Here's how the part is built. I have some questions about the finished solid (model axes, mm). Coordinates: 2 decimals unless noted, no trailing zeros. Loops run counter-clockwise (first coordinate to the right, second up) from the corner with the lowest first, then second, coordinate; pieces in that order, holes last. Notation, with made-up numbers: (44.5, 71.5) -> (90.5, 71.5) arc R18 cw to (90.5, 84.5) -> close; hole circle Ø9 at (-9, 27). An arc over 180 degrees is marked (long way). Use CSV: the item, a comma, the result in double quotes. Start each with the question number.
from build123d import *

# Parameters (mm, degrees)
SKETCH1_R           = 6.5
BOSS_EXTRUDE1_DEPTH = 4
SKETCH5_R           = 1.5
CUT_EXTRUDE1_DEPTH  = 4


with BuildPart() as part:
    # Sketch1 → Boss-Extrude1 (new body)
    with BuildSketch(Plane.XY):
        Circle(SKETCH1_R)
    extrude(amount=BOSS_EXTRUDE1_DEPTH)

    # Sketch4 → Cut-Revolve1 (revolve, cut)
    with BuildSketch(Plane(origin=(0, 0, 0), x_dir=(0, -1, 0), z_dir=(1, 0, 0)), mode=Mode.PRIVATE) as cut_revolve1_sk:
        with BuildLine():
            Line((6.5, -1), (6.5, -3))
            ThreePointArc((6.5, -3), (5.5, -2), (6.5, -1))
        make_face()
    revolve(cut_revolve1_sk.sketch.rotate(Axis((0, 0, 0), (0, 0, 1)), 270), axis=Axis((0, 0, 0), (0, 0, 1)), mode=Mode.SUBTRACT)

    # Sketch5 → Cut-Extrude1 (cut)
    with BuildSketch(Plane(origin=(0, 0, 0), x_dir=(-1, 0, 0), z_dir=(0, 0, -1))):
        Circle(SKETCH5_R)
    extrude(amount=-CUT_EXTRUDE1_DEPTH, mode=Mode.SUBTRACT)


solid = part.part
1) Thinking about a two-plate mould opening in Y: for faces 1 (the face through (0, 2, 4)), 2 (the face through (1.5, 0.07, 1.97)), 3 (the face through (-5.158, -3.955, 3.493)), which applies, pulls with the +Y half, pulls with the -Y half, needs draft (parallel to the pull), parting line crosses it, or undercut?
2) Please list where these lines run through material, in increasing order: L1, parallel to Z at x = 5, y = -3.25; L2, parallel to Y at x = 0, z = 1.6; L3, parallel to Y at x = 0, z = 2.15. Write a range as [from, to].
3) For P1, Ø2, axis at y = 3, z = 2.5, coming from the -X side; P2, Ø1, axis at x = 2.5, y = 1.5, coming from the -Z side; P3, Ø1.8, axis at x = 0, y = 0, coming from the -Z side; P4, Ø1.5, axis at x = 4, z = 1.5, coming from the +Y side, each with a flat end and sliding along its axis, tell me the tip position at first contact or that it passes through.
4) I want a section at D-D, the plane z = 1.25. Please give me the cut outline in (x, y).
5) I want a section at C-C, the plane z = 3.4. Please give me the cut outline in (x, y).
6) I want a section at A-A, the plane x = 0. Please give me the cut outline in (y, z), plus the area to 3 significant figures.
Return value:
1,face 1,"needs draft"
1,face 2,"undercut"
1,face 3,"parting line crosses it"
2,L1,"z = [0, 1.16], [2.84, 4]"
2,L2,"y = [-5.58, -1.5], [1.5, 5.58]"
2,L3,"y = [-5.51, -1.5], [1.5, 5.51]"
3,P1,"stops at x = -6.14"
3,P2,"stops at z = 0"
3,P3,"passes through"
3,P4,"stops at y = 5.51"
4,outline,"circle Ø11.68 at (0, 0); hole circle Ø3 at (0, 0)"
5,outline,"circle Ø13 at (0, 0); hole circle Ø3 at (0, 0)"
6,outline,"(-6.5, 0) -> (-1.5, 0) -> (-1.5, 4) -> (-6.5, 4) -> (-6.5, 3) arc R1 cw to (-6.5, 1) -> close; (1.5, 0) -> (6.5, 0) -> (6.5, 1) arc R1 cw to (6.5, 3) -> (6.5, 4) -> (1.5, 4) -> close"
6,area,"36.9 mm²"
